Check sheet for the drawn part. Datum: minimum x, y, z corner. Units: mm. A direction names the side the tool comes from. Round coordinates to 2 decimals unless told otherwise and drop trailing zeros. Write each loop counter-clockwise with the first axis right and the second up, starting at its lowest first coordinate (ties: lowest second). Pieces come first, ordered by that corner, then holes.
Item 1: Cross-section at B-B on z = 14.15. Enter the section's corners in (x, y).
Item 2: Cross-section at A-A on y = 12. Enter the section's corners in (x, z), plus the area to 3 significant figures.
Item 3: Go/stop test with flat-tipped pins: pin 1 Ø0.8 at (y, z) = (24, 27.5) entering from -X; pin 2 Ø4.5 at (y, z) = (24, 14.15) entering from -X; pin 3 Ø3 at (y, z) = (18, 20.15) entering from +X; pin 4 Ø4 at (x, z) = (37, 5.5) entering from +Y. Record where each tip stops, or that it passes through.
Item 4: Release check for a two-part mould opening along X. For the marked faces 3, 4, 5 and 6 record: +X half, -X half, draft (parallel to the pull), parting line (faces both ways), or undercut.
Item 5: Cross-section at D-D on y = 18. Enter the section's corners in (x, z).
Item 6: Cross-section at C-C on x = 11.15. Enter the section's corners in (y, z).
Item 7: Material ranges on line 1 (X direction, y = 1.4, z = 14.15); line 2 (Y direction, x = 63.4, z = 14.15); line 3 (Z direction, x = 11.15, y = 2.45), recorded low to high.
Item 8: Tool access check on the marked faces 1 and 2. Record the directions out of +Z, -Z, +X, -X, +Y, -Y that give a thin tool (end or side, any length) a straight path to the whole face; none if there is none.
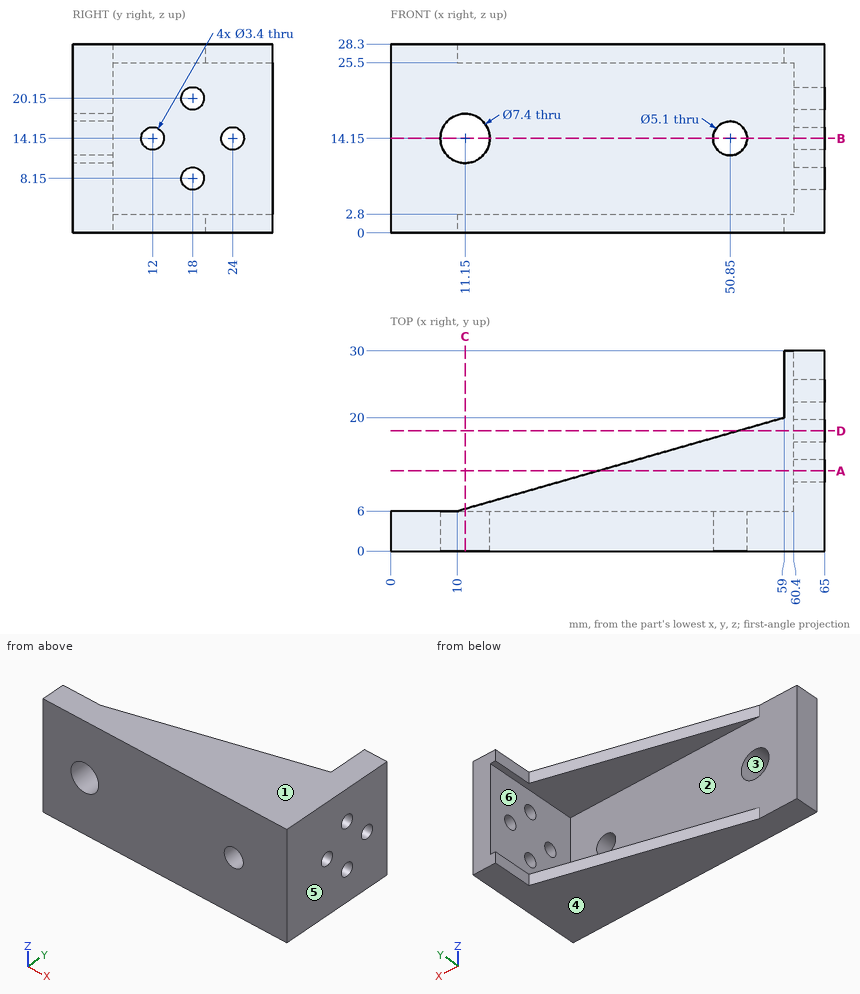
Response values:
1. outline: (0, 0) - (7.45, 0) - (7.45, 6) - (0, 6) - close; (14.85, 0) - (48.3, 0) - (48.3, 6) - (14.85, 6) - close; (53.4, 0) - (65, 0) - (65, 10.3) - (60.4, 10.3) - (60.4, 6) - (53.4, 6) - close; (60.4, 13.7) - (65, 13.7) - (65, 22.3) - (60.4, 22.3) - close; (60.4, 25.7) - (65, 25.7) - (65, 30) - (60.4, 30) - close
2. outline: (31, 0) - (65, 0) - (65, 12.45) - (60.4, 12.45) - (60.4, 2.8) - (31, 2.8) - close; (31, 25.5) - (60.4, 25.5) - (60.4, 15.85) - (65, 15.85) - (65, 28.3) - (31, 28.3) - close
2. area: 279 mm2
3. pin 1: stops at x = 59
3. pin 2: stops at x = 60.4
3. pin 3: passes through
3. pin 4: stops at y = 6
4. face 3: undercut
4. face 4: draft
4. face 5: +X half
4. face 6: -X half
5. outline: (52, 0) - (65, 0) - (65, 6.45) - (60.4, 6.45) - (60.4, 2.8) - (52, 2.8) - close; (52, 25.5) - (60.4, 25.5) - (60.4, 21.85) - (65, 21.85) - (65, 28.3) - (52, 28.3) - close; (60.4, 9.85) - (65, 9.85) - (65, 18.45) - (60.4, 18.45) - close
6. outline: (0, 0) - (6.33, 0) - (6.33, 2.8) - (6, 2.8) - (6, 10.45) - (0, 10.45) - close; (0, 17.85) - (6, 17.85) - (6, 25.5) - (6.33, 25.5) - (6.33, 28.3) - (0, 28.3) - close
7. line 1: x = 0 to 7.45, 14.85 to 48.3, 53.4 to 65
7. line 2: y = 0 to 10.3, 13.7 to 22.3, 25.7 to 30
7. line 3: z = 0 to 10.45, 17.85 to 28.3
8. face 1: +Z, +X, -X, +Y, -Y
8. face 2: -X, +Y
